from build123d import *

# Parameters (mm, degrees)
SKETCH1_W           = 139.7
SKETCH1_H           = 76.2
BOSS_EXTRUDE1_DEPTH = 6.35
SKETCH2_W           = 139.7
SKETCH2_H           = 12.7
BOSS_EXTRUDE2_DEPTH = 19.05
SKETCH3_R           = 2.032
CUT_EXTRUDE1_DEPTH  = 82.814026915
CUT_EXTRUDE2_DEPTH  = 3.048


with BuildPart() as part:
    # Sketch1 → Boss-Extrude1 (new body)
    with BuildSketch(Plane(origin=(0, 0, 0), x_dir=(1, 0, 0), z_dir=(0, 1, 0))):
        Rectangle(SKETCH1_W, SKETCH1_H)
    extrude(amount=BOSS_EXTRUDE1_DEPTH)

    # Sketch2 → Boss-Extrude2 (add)
    with BuildSketch(Plane(origin=(0, 6.35, 0), x_dir=(1, 0, 0), z_dir=(0, 1, 0))):
        with Locations((0, -31.75)):
            Rectangle(SKETCH2_W, SKETCH2_H)
    extrude(amount=BOSS_EXTRUDE2_DEPTH)

    # Sketch3 → Cut-Extrude1 (cut, through all)
    with BuildSketch(Plane(origin=(0, 6.35, 0), x_dir=(1, 0, 0), z_dir=(0, 1, 0))):
        with Locations(Location((-53.34, -21.59, 0), (0, 0, 270))):
            Circle(SKETCH3_R)
    extrude(amount=-CUT_EXTRUDE1_DEPTH, mode=Mode.SUBTRACT)

    # Sketch4 → Cut-Extrude2 (cut)
    with BuildSketch(Plane.XZ):
        Polygon((-50.927, 25.769438599), (-55.753, 25.769438599), (-58.166, 21.59), (-55.753, 17.410561401), (-50.927, 17.410561401), (-48.514, 21.59), align=None)
    extrude(amount=-CUT_EXTRUDE2_DEPTH, mode=Mode.SUBTRACT)


solid = part.part
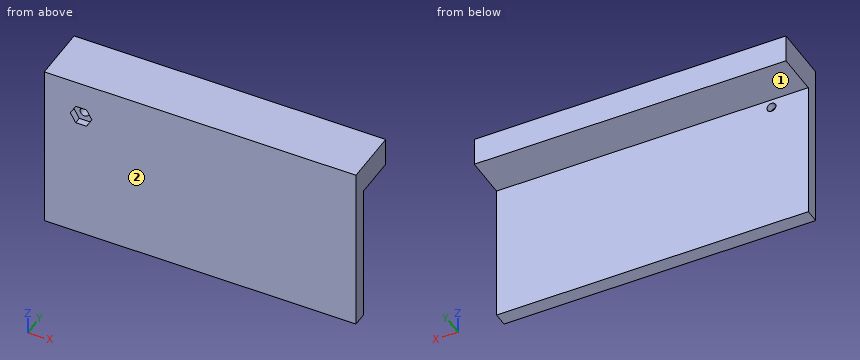
Work out the finished part from the listing and answer in its coordinate system (mm). Face numbers are marked on the shaded views. A direction names the side the tool comes from. Give positions to 0.01 mm unless a question says otherwise; leave off trailing zeros. Order: outer loops, then holes, each group sorted by start corner. A loop starts at its lowest first (then second) coordinate and runs counter-clockwise, first axis right, second up. Notation, with made-up numbers: M 53,-36.75 L 90,-36.75 A22 cw 90,-26.75 Z; hole C 33.5,-20.5 d7. An arc over 180 degrees is marked long. Return JSON: item names as keys, results as strings.
Q1. Find the intervals of material crossed by line 1 along X through (y, z) = (4.65, 21.59); line 2 along Y through (x, z) = (-43, 19); line 3 along Z through (x, y) = (-45.5, 24.25), in increasing order. Write a range as [from, to].
Answer below:
{"line 1": "x = [-69.85, -55.37], [-51.31, 69.85]", "line 2": "y = [0, 6.35]", "line 3": "z = [25.4, 38.1]"}
Q2. Find section C-C, the plane z = -6.5. Write down the section's boundary in (x, y), and give its area (3 significant figures).
Answer below:
{"outline": "M -69.85,0 L 69.85,0 L 69.85,6.35 L -69.85,6.35 Z", "area": "887 mm^2"}
Q3. Find section B-B, the plane x = -37.5. Write down the section's boundary in (y, z).
Answer below:
{"outline": "M 0,-38.1 L 6.35,-38.1 L 6.35,25.4 L 25.4,25.4 L 25.4,38.1 L 0,38.1 Z"}
Q4. Find section A-A, the plane x = -53.34. Write down the section's boundary in (y, z).
Answer below:
{"outline": "M 0,-38.1 L 6.35,-38.1 L 6.35,19.56 L 3.05,19.56 L 3.05,17.41 L 0,17.41 Z; M 0,25.77 L 3.05,25.77 L 3.05,23.62 L 6.35,23.62 L 6.35,25.4 L 25.4,25.4 L 25.4,38.1 L 0,38.1 Z"}
Q5. Each of these flat-tipped pins is pushed along its axis until it touches: pin 1 (1 mm diameter, centred on y = 8, z = 11, fed in from -X) (1 decimal); pin 2 (1 mm diameter, centred on x = -1.5, z = -5.5, fed in from +Y); pin 3 (6 mm diameter, centred on x = -33.5, y = 17, fed in from -Z). Where does it stop, or does it pass through?
Answer below:
{"pin 1": "passes through", "pin 2": "stops at y = 6.35", "pin 3": "stops at z = 25.4"}
Q6. Which of the six approach directions +Z, -Z, +X, -X, +Y, -Y give full straight-line access (tool end or side, diameter ignored) to the marked faces 1 and 2?
Answer below:
{"face 1": "-Z, +X, -X, +Y", "face 2": "+Z, -Z, +X, -X, -Y"}
